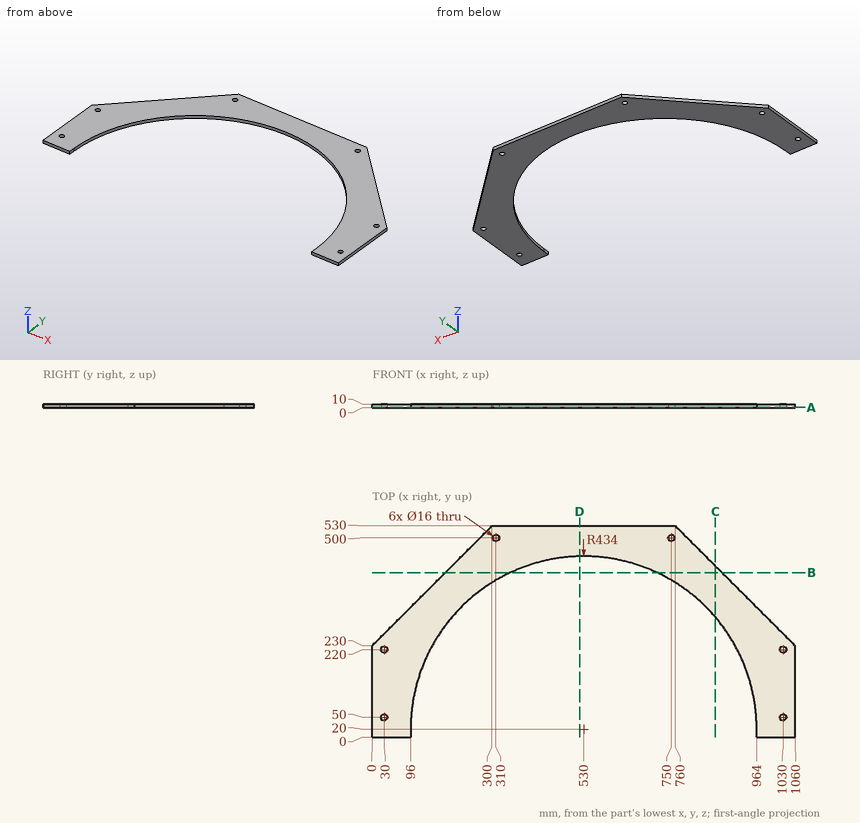
Job drawing, mm, ordinate dimensions from the low corner. One solid piece. Give positions to 0.01 mm unless a question says otherwise; leave off trailing zeros. Order: outer loops, then holes, each group sorted by start corner. A loop starts at its lowest first (then second) coordinate and runs counter-clockwise, first axis right, second up. Notation, with made-up numbers: M 19,10.25 L 47,10.25 A24 cw 47,36.25 Z; hole C -24,-33 d11. An arc over 180 degrees is marked long. Put each result on its own line as item: value. Start each with the question number.
(1) Band-saw the part on D-D on x = 520. Give the cut face in (y, z).
(2) Drill centre lines: L1, parallel to X at y = 55.5, z = 4.25; L2, parallel to X at y = 284, z = 3.5; L3, parallel to X at y = 197.5, z = 8. Where is each one in solid material? Low to high. Write a range as [from, to].
(3) Band-saw the part on B-B on y = 413. Give the cut face in (x, z), then the cut area to 3 significant figures.
(4) Pin check, flat tips, straight feed: pin 1 Ø13 at (x, y) = (30, 220) entering from +Z; pin 2 Ø1 at (x, z) = (367, 6.5) entering from -Y; pin 3 Ø2 at (x, z) = (357.5, 2) entering from -Y. Stop position of each tip, or through.
(5) Band-saw the part on C-C on x = 860. Give the cut face in (y, z).
(6) Band-saw the part on A-A on z = 1.5. Give the cut face in (x, y).
Results below:
1. outline: M 453.88,0 L 530,0 L 530,10 L 453.88,10 Z
2. L1: x = [0, 24.19], [35.81, 97.45], [962.55, 1024.19], [1035.81, 1060]
2. L2: x = [54, 185.53], [874.47, 1006]
2. L3: x = [0, 133.96], [926.04, 1060]
3. outline: M 183,0 L 345.86,0 L 345.86,10 L 183,10 Z; M 714.14,0 L 877,0 L 877,10 L 714.14,10 Z
3. area: 3,260 mm2
4. pin 1: passes through
4. pin 2: stops at y = 422.02
4. pin 3: stops at y = 417.81
5. outline: M 301.88,0 L 430,0 L 430,10 L 301.88,10 Z
6. outline: M 0,0 L 96,0 L 96,20 A434 cw 964,20 L 964,0 L 1060,0 L 1060,230 L 760,530 L 300,530 L 0,230 Z; hole C 30,50 d16; hole C 30,220 d16; hole C 310,500 d16; hole C 750,500 d16; hole C 1030,50 d16; hole C 1030,220 d16
